CAD build for the part. Positions are in the model's coordinates, mm. A direction names the side the tool comes from. Give positions to 0.01 mm unless a question says otherwise; leave off trailing zeros. Write each loop counter-clockwise with the first axis right and the second up, starting at its lowest first coordinate (ties: lowest second). Pieces come first, ordered by that corner, then holes. Notation, with made-up numbers: (54, -16) -> (67, -16) arc R18 cw to (67, -6) -> close; hole circle Ø4 at (52, 15.5). An arc over 180 degrees is marked (long way). Answer as a JSON object with one key per item and string values.
Autodesk Inventor part; units mm, degrees
ref_plane "YZ Plane" through (0, 0, 0) normal (1, 0, 0) x (0, 1, 0)
ref_plane "XZ Plane" through (0, 0, 0) normal (0, 1, 0) x (-1, 0, 0)
ref_plane "XY Plane" through (0, 0, 0) normal (0, 0, 1) x (1, 0, 0)
sketch "Skizze2" plane through (0, 0, 0) normal (0, 0, 1) x (1, 0, 0)
  line L0 (-5, 7) -> (5, 7)
  line L1 (5, 7) -> (5, -7)
  line L2 (5, -7) -> (-5, -7)
  line L3 (-5, -7) -> (-5, 7)
  line L4 (0, 9.8) -> (0, -9.8)
  line L5 (-7, 0) -> (7, 0)
  point P0 (0, 0)
  point P1 (-5, 0)
  point P2 (0, 7)
  dimension "d0" = 14
  dimension "d1" = 10
extrude "Extrusion1" add sketch "Skizze2" along normal blind 3.5
sketch "Skizze3" plane through (0, 0, 3.5) normal (0, 0, 1) x (1, 0, 0)
  line L0 (5, -7) -> (5, 7)
  line L1 (5, 7) -> (-5, 7)
  line L2 (-5, 7) -> (-5, -7)
  line L3 (-5, -7) -> (5, -7)
  line L4 (5, 7) -> (-5, 7)
  line L5 (-5, 7) -> (-5, 5.5)
  line L6 (-5, 5.5) -> (5, 5.5)
  line L7 (5, 5.5) -> (5, 7)
  line L8 (-5, 7) -> (-5, -7)
  line L9 (-5, -7) -> (5, -7)
  line L10 (5, -7) -> (5, -5.5)
  line L11 (5, -5.5) -> (-5, -5.5)
  line L12 (-5, -5.5) -> (-5, -7)
  point P0 (0, 0)
  dimension "d4" = 1.5
  dimension "d5" = 1.5
extrude "Extrusion2" add sketch "Skizze3" along normal blind 1 contours L3 L2 L11 L0 | L6 L2 L1 L0
sketch "Skizze4" plane through (0, 0, 0) normal (0, 0, -1) x (-1, 0, 0)
  line L0 (5, -7) -> (-5, -7)
  line L1 (5, -7) -> (-5, -7)
  line L2 (-5, -7) -> (-5, -15)
  line L3 (-5, -15) -> (5, -15)
  line L4 (5, -15) -> (5, -7)
  line L5 (-5, 7) -> (5, 7)
  line L6 (5, 7) -> (5, 15)
  line L7 (5, 15) -> (-5, 15)
  line L8 (-5, 15) -> (-5, 7)
  line L9 (5, -7) -> (-5, -7)
  line L10 (-5, 7) -> (5, 7)
  line L11 (5, 7) -> (5, -7)
  line L12 (-5, -7) -> (-5, 7)
  line L13 (5, 5.5) -> (5, -5.5)
  point P0 (0, 0)
  point P1 (-5, -7)
  point P2 (0, -15)
  point P3 (0, -11)
  point P4 (0, 11)
  point P5 (5, -11)
  point P6 (5, 11)
  dimension "d8" = 8
  dimension "d9" = 8
  dimension "d31" = 10
  dimension "d32" = 22
extrude "Extrusion3" add sketch "Skizze4" against normal up to surface (4.5 mm away) contours L4 L3 L2 L0 | L8 L7 L6 L5
sketch "Skizze5" plane through (0, 0, 0) normal (0, 0, -1) x (-1, 0, 0)
  line L0 (-5, 5.5) -> (-5, 15)
  line L1 (-5, -5.5) -> (-5, -15)
  line L2 (-5, -15) -> (5, -15)
  line L3 (5, 15) -> (-5, 15)
  line L4 (-7, 0) -> (7, 0)
  point P0 (0, 11.25)
  point P1 (0, -11.25)
  point P2 (0, -15)
  point P3 (0, 15)
  dimension "d39" = 22.5
  dimension "d40" = 11.25
hole "Bohrung1" at (0, -11.25, 0) direction (0, 0, 1) diameter 5.2 end through all
fillet "Rundung1" radius 3 4 edges at (-5, -15, 2.25) (5, -15, 2.25) (5, 15, 2.25) (-5, 15, 2.25)
pattern_linear "Rechteckige Anordnung1" count 2 spacing 22.5 along (0, 1, 0) of "Bohrung1"
equation "\"d5\" = d4"
equation "\"d9\" = d8"
equation "\"d24\" = d34"
properties part number "LED_Strip_Halter_einzeln" material "PA 6 schwarz"
1) Slice it at C-C (z = 0.65). List the corners of the cut face in (x, y).
Model answer:
{"outline": "(-5, -12) arc R3 ccw to (-2, -15) -> (2, -15) arc R3 ccw to (5, -12) -> (5, 12) arc R3 ccw to (2, 15) -> (-2, 15) arc R3 ccw to (-5, 12) -> close; hole circle Ø5.2 at (0, -11.25); hole circle Ø5.2 at (0, 11.25)"}
2) Mould opens along X. For faces 3 (the cylindrical face through (-0.78, -8.77, 2.28)), 4 (the flat face through (5, 0, 2)), 5 (the flat face through (0, 5.5, 4)) say: released by +X, released by -X, zero draft, split by the parting line, or undercut.
Model answer:
{"face 3": "undercut", "face 4": "released by +X", "face 5": "zero draft"}
3) Slice it at D-D (y = 3.25). List the corners of the cut face in (x, z).
Model answer:
{"outline": "(-5, 0) -> (5, 0) -> (5, 3.5) -> (-5, 3.5) -> close"}
4) Wall check: probe 1 along Y at (x, z) = (0, 3.2); probe 2 along Y at (x, z) = (2.25, 2.4); probe 3 along Y at (x, z) = (1, 4.1). Give the ranges that are in metal, low to high.
Model answer:
{"probe 1": "y = -15 to -13.85, -8.65 to 8.65, 13.85 to 15", "probe 2": "y = -14.99 to -12.55, -9.95 to 9.95, 12.55 to 14.99", "probe 3": "y = -15 to -13.65, -8.85 to -5.5, 5.5 to 8.85, 13.65 to 15"}
5) Slice it at B-B (y = -11.25). List the corners of the cut face in (x, z), then the cut area to 3 significant figures.
Model answer:
{"outline": "(-5, 0) -> (-2.6, 0) -> (-2.6, 4.5) -> (-5, 4.5) -> close; (2.6, 0) -> (5, 0) -> (5, 4.5) -> (2.6, 4.5) -> close", "area": "21.6 mm2"}
6) 3-axis set-ups, long thin cutter, end or side, ignore diameter. For faces 1 (the flat face through (0, 15, 2)), 2 (the flat face through (0, -5.5, 4)): which of +Z, -Z, +X, -X, +Y, -Y reach the whole face in a straight line?
Model answer:
{"face 1": "+Z, -Z, +X, -X, +Y", "face 2": "+Z, +X, -X"}
7) Pin check, flat tips, straight feed: pin 1 (4.5 mm diameter, centred on x = 0, y = -11.25, fed in from +Z); pin 2 (2 mm diameter, centred on x = -3, z = 3, fed in from +Y); pin 3 (5 mm diameter, centred on x = -2.5, y = 0, fed in from +Z). Stop position of each tip, or through.
Model answer:
{"pin 1": "passes through", "pin 2": "stops at y = 15", "pin 3": "stops at z = 3.5"}
8) Slice it at A-A (x = 0). List the corners of the cut face in (y, z).
Model answer:
{"outline": "(-15, 0) -> (-13.85, 0) -> (-13.85, 4.5) -> (-15, 4.5) -> close; (-8.65, 0) -> (8.65, 0) -> (8.65, 4.5) -> (5.5, 4.5) -> (5.5, 3.5) -> (-5.5, 3.5) -> (-5.5, 4.5) -> (-8.65, 4.5) -> close; (13.85, 0) -> (15, 0) -> (15, 4.5) -> (13.85, 4.5) -> close"}
